from build123d import *

# Parameters (mm, degrees)
F1_DEPTH = 63.5
F2_DEPTH = 50.8


with BuildPart() as f1:
    # F0 (on Front) → F1 (new body, symmetric)
    with BuildSketch(Plane.XZ):
        Polygon((-41.275, 9.525), (-41.275, -9.525), (41.275, -9.525), (41.275, 9.525), (22.4790014327, 9.525), align=None)
    extrude(amount=F1_DEPTH, both=True)

    # F0 (on Front) → F2 (join)
    with BuildSketch(Plane.XZ):
        Polygon((-41.275, 9.525), (-41.275, -9.525), (41.275, -9.525), (41.275, 9.525), (22.4790014327, 9.525), align=None)
        with BuildLine():
            add(Edge.make_bspline(
                [(-41.275, 9.525), (-35.7326114907, 63.6337083014), (19.6466617219, 65.4086383739), (63.8208144069, 64.4769455383)],
                knots=[0, 0, 0, 0, 117.4701032347, 117.4701032347, 117.4701032347, 117.4701032347], degree=3))
            Line((-41.275, 9.525), (22.4790014327, 9.525))
            Line((22.4790014327, 9.525), (22.4790014327, 47.0458286018))
            ThreePointArc((22.4790014327, 47.0458286018), (28.8618939863, 60.471876969), (43.3038324118, 63.9975693303))
            Line((43.3038324118, 63.9975693303), (63.8208144069, 63.9975693303))
            Line((63.8208144069, 63.9975693303), (63.8208144069, 64.4769455383))
        make_face()
        with BuildLine():
            Line((22.4790014327, 9.525), (41.275, 9.525))
            Line((41.275, 9.525), (41.275, 28.575))
            ThreePointArc((41.275, 28.575), (45.9246798487, 39.8003201513), (57.15, 44.45))
            Line((57.15, 44.45), (63.8208144069, 44.45))
            Line((63.8208144069, 44.45), (63.8208144069, 63.9975693303))
            Line((63.8208144069, 63.9975693303), (43.3038324118, 63.9975693303))
            ThreePointArc((43.3038324118, 63.9975693303), (28.8618939863, 60.471876969), (22.4790014327, 47.0458286018))
            Line((22.4790014327, 47.0458286018), (22.4790014327, 9.525))
        make_face()
        with BuildLine():
            add(Edge.make_bspline(
                [(63.8208144069, 64.4769455383), (71.9097851364, 64.3063381669), (79.6230338842, 64.0449742774), (86.5857569244, 63.9975693303)],
                knots=[117.4701032347, 117.4701032347, 117.4701032347, 117.4701032347, 138.9806963961, 138.9806963961, 138.9806963961, 138.9806963961], degree=3))
            Line((63.8208144069, 64.4769455383), (63.8208144069, 63.9975693303))
            Line((63.8208144069, 63.9975693303), (86.5857569244, 63.9975693303))
        make_face()
        with BuildLine():
            Line((63.8208144069, 66.675), (63.8208144069, 64.4769455383))
            add(Edge.make_bspline(
                [(63.8208144069, 64.4769455383), (71.9097851364, 64.3063381669), (79.6230338842, 64.0449742774), (86.5857569244, 63.9975693303)],
                knots=[117.4701032347, 117.4701032347, 117.4701032347, 117.4701032347, 138.9806963961, 138.9806963961, 138.9806963961, 138.9806963961], degree=3))
            Line((86.5857569244, 63.9975693303), (85.725, 44.45))
            Line((85.725, 44.45), (63.8208144069, 44.45))
            Line((63.8208144069, 44.45), (63.8208144069, 38.1))
            Line((63.8208144069, 38.1), (114.6208144069, 38.1))
            Line((114.6208144069, 38.1), (114.6208144069, 66.675))
            Line((114.6208144069, 66.675), (63.8208144069, 66.675))
        make_face()
        Polygon((86.5857569244, 63.9975693303), (63.8208144069, 63.9975693303), (63.8208144069, 44.45), (85.725, 44.45), align=None)
    extrude(amount=F2_DEPTH)


solid = f1.part
Could you check a few things on this model? Use its own coordinates, in mm. A direction names the side the tool comes from. Coordinates: 2 decimals unless noted, no trailing zeros. Loops run counter-clockwise (first coordinate to the right, second up) from the corner with the lowest first, then second, coordinate; pieces in that order, holes last.
1. For P1, Ø1, axis at x = 85, z = 45, coming from the -Y side; P2, Ø19, axis at x = -15, y = 25, coming from the +Z side (3 decimals); P3, Ø1.5, axis at y = -10.5, z = 27.5, coming from the -X side, each with a flat end and sliding along its axis, tell me the tip position at first contact or that it passes through.
2. For faces 1 (the face through (41.275, 1, 5)), 2 (the face through (1, 31, 9.525)), 3 (the face through (45.802, -25.044, 39.676)), which set-ups out of +Z, -Z, +X, -X, +Y, -Y let a thin tool reach every point of the face, with its end or its side?
3. Imagine slicing it at A-A (z = -2). Please give me the cut outline in (x, y) (3 decimals), and give its area (3 significant figures).
4. I need wall thicknesses on L1, parallel to X at y = 35, z = -5 (3 decimals); L2, parallel to Y at x = 13, z = 39.5; L3, parallel to Z at x = -31, y = 31 (3 decimals). Which ranges of each line are inside material? Lowest first, please.
5. Imagine slicing it at B-B (y = 21.5). Please give me the cut outline in (x, z) (3 decimals), and give its area (3 significant figures).
Computed values:
1. P1: stops at y = -50.8
1. P2: stops at z = 9.525
1. P3: stops at x = -37.26
2. face 1: -Z, +X, +Y, -Y
2. face 2: +Z, +X, -X, +Y
2. face 3: -Z, +Y, -Y
3. outline: (-41.275, -63.5) - (41.275, -63.5) - (41.275, 63.5) - (-41.275, 63.5) - close
3. area: 10,500 mm2
4. L1: x = -41.275 to 41.275
4. L2: y = -50.8 to 0
4. L3: z = -9.525 to 9.525
5. outline: (-41.275, -9.525) - (41.275, -9.525) - (41.275, 9.525) - (-41.275, 9.525) - close
5. area: 1,570 mm2
